Read the model definition and answer for the solid it produces. Units are mm, in the model's axes. Face numbers are marked on the shaded views. Give positions to 0.01 mm unless a question says otherwise; leave off trailing zeros. Write each loop counter-clockwise with the first axis right and the second up, starting at its lowest first coordinate (ties: lowest second). Pieces come first, ordered by that corner, then holes. Notation, with made-up numbers: M 46,2.25 L 84,2.25 A27 cw 84,38.25 Z; hole C 87.5,-11 d7. An arc over 180 degrees is marked long. Use a Markdown table: item, result. Add a question column.
Item 1: A cutting plane is placed at C-C on x = 5. Determine the outline of the cut face in (y, z) (3 decimals), then the cut area to 3 significant figures.
Item 2: A cutting plane is placed at B-B on z = -1.45. Determine the outline of the cut face in (x, y) (3 decimals).
Item 3: A cutting plane is placed at A-A on x = -2.54. Determine the outline of the cut face in (y, z) (3 decimals), then the cut area to 3 significant figures.
Item 4: A cutting plane is placed at D-D on y = 7.25. Determine the outline of the cut face in (x, z), then the cut area to 3 significant figures.
Item 5: Consider probe 1 along Y at (x, z) = (0, -0.8) (3 decimals); probe 2 along X at (y, z) = (-5.5, -1.3) (3 decimals); probe 3 along X at (y, z) = (7.5, -0.25). Determine where each line is inside the solid, lowest interval first. Write a range as [from, to].
Item 6: The mould has two halves that part along X. Classify the marked faces 1, 2, 3 and 4: pulls with the +X half, pulls with the -X half, needs draft (parallel to the pull), parting line crosses it, or undercut.
Item 7: Given P1, Ø2, axis at x = -5.715, y = 5.715, coming from the -Z side, flat-ended and moving along its own axis, determine where the tip first touches the part or whether it passes through.
from build123d import *

# Parameters (mm, degrees)
PAD018_DEPTH           = 1.65
SKETCH050_R            = 1.27
POCKET030_DEPTH        = 1.651
SKETCH051_R            = 0.4
POCKET029_DEPTH        = 1.651
LINEARPATTERN004_COUNT = 3
LINEARPATTERN004_PITCH = 2.54
LINEARPATTERN005_COUNT = 3
LINEARPATTERN005_PITCH = 2.54


with BuildPart() as part:
    # Sketch049 → Pad018 (new body)
    with BuildSketch(Plane.XY):
        with BuildLine():
            Line((-5.715, 8.255), (5.715, 8.255))
            ThreePointArc((8.255, 5.715), (7.511051, 7.511051), (5.715, 8.255))
            Line((8.255, 5.715), (8.255, -5.715))
            ThreePointArc((5.715, -8.255), (7.511051, -7.511051), (8.255, -5.715))
            Line((5.715, -8.255), (-5.715, -8.255))
            ThreePointArc((-8.255, -5.715), (-7.511051, -7.511051), (-5.715, -8.255))
            Line((-8.255, -5.715), (-8.255, 5.715))
            ThreePointArc((-5.715, 8.255), (-7.511051, 7.511051), (-8.255, 5.715))
        make_face()
    extrude(amount=-PAD018_DEPTH)

    # Sketch050 → Pocket030 (cut, through all)
    with BuildSketch(Plane.XY):
        with Locations((-5.715, 5.715)):
            Circle(SKETCH050_R)
        with Locations((5.715, 5.715)):
            Circle(SKETCH050_R)
    extrude(amount=-POCKET030_DEPTH, mode=Mode.SUBTRACT)

    # Sketch051 → Pocket029 (cut, through all)
    with BuildSketch(Plane.XY):
        with Locations((0, -5.715)):
            Circle(SKETCH051_R)
    pocket029 = extrude(amount=-POCKET029_DEPTH, mode=Mode.SUBTRACT)

    # LinearPattern004: Pocket029 ×3
    with Locations(*[(i * LINEARPATTERN004_PITCH, 0, 0) for i in range(1, LINEARPATTERN004_COUNT)]):
        add(pocket029, mode=Mode.SUBTRACT)

    # LinearPattern005: Pocket029 ×3
    with Locations(*[(-i * LINEARPATTERN005_PITCH, 0, 0) for i in range(1, LINEARPATTERN005_COUNT)]):
        add(pocket029, mode=Mode.SUBTRACT)


solid = part.part
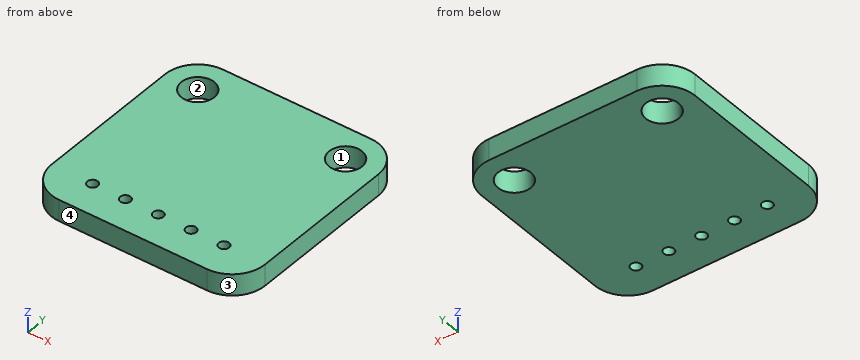
Filled in:
| question | item | result |
|---|---|---|
| 1 | outline | M -8.255,-1.65 L -6.107,-1.65 L -6.107,0 L -8.255,0 Z; M -5.323,-1.65 L 4.665,-1.65 L 4.665,0 L -5.323,0 Z; M 6.765,-1.65 L 8.255,-1.65 L 8.255,0 L 6.765,0 Z |
| 1 | area | 22.5 mm² |
| 2 | outline | M -8.255,-5.715 A2.54 ccw -5.715,-8.255 L 5.715,-8.255 A2.54 ccw 8.255,-5.715 L 8.255,5.715 A2.54 ccw 5.715,8.255 L -5.715,8.255 A2.54 ccw -8.255,5.715 Z; hole C -5.715,5.715 d2.54; hole C -5.08,-5.715 d0.8; hole C -2.54,-5.715 d0.8; hole C 0,-5.715 d0.8; hole C 2.54,-5.715 d0.8; hole C 5.715,5.715 d2.54; hole C 5.08,-5.715 d0.8 |
| 3 | outline | M -8.255,-1.65 L -6.115,-1.65 L -6.115,0 L -8.255,0 Z; M -5.315,-1.65 L 8.255,-1.65 L 8.255,0 L -5.315,0 Z |
| 3 | area | 25.9 mm² |
| 4 | outline | M -7.74,-1.65 L 7.74,-1.65 L 7.74,0 L -7.74,0 Z |
| 4 | area | 25.5 mm² |
| 5 | probe 1 | [-8.255, -6.115], [-5.315, 8.255] |
| 5 | probe 2 | [-8.255, -5.417], [-4.743, -2.877], [-2.203, -0.337], [0.337, 2.203], [2.877, 4.743], [5.417, 8.255] |
| 5 | probe 3 | [-7.52, 7.52] |
| 6 | face 1 | undercut |
| 6 | face 2 | undercut |
| 6 | face 3 | pulls with the +X half |
| 6 | face 4 | needs draft |
| 7 | P1 | through |
